Could you check a few things on this model? Use its own coordinates, in mm. Face numbers are marked on the shaded views. Give positions to 0.01 mm unless a question says otherwise; leave off trailing zeros. Loops run counter-clockwise (first coordinate to the right, second up) from the corner with the lowest first, then second, coordinate; pieces in that order, holes last. Notation, with made-up numbers: (65, 77.5) - (109, 77.5) arc R19 ccw to (109, 83.5) - close; hole circle Ø4 at (64, 0.25). An arc over 180 degrees is marked (long way). Write each question's results on one line, items separated by ' | '. Start each with the question number.
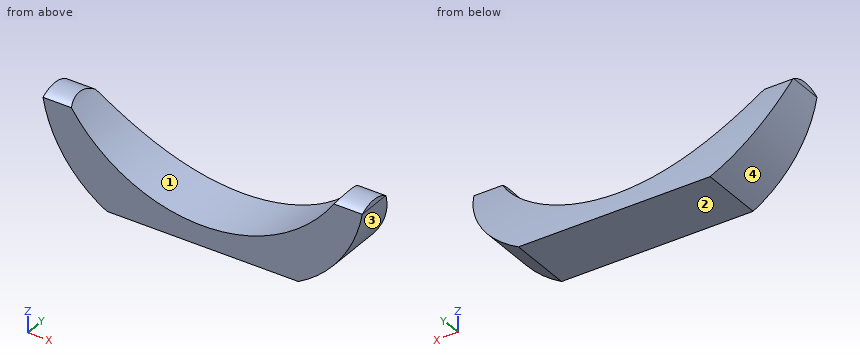
```python
from build123d import *

# Parameters (mm, degrees)
SKETCH2_W           = 500
SKETCH2_H           = 150
BOSS_EXTRUDE1_DEPTH = 100
CUT_EXTRUDE1_DEPTH  = 540
SKETCH5_R           = 249.318658331
CUT_EXTRUDE2_DEPTH  = 560
CUT_EXTRUDE3_DEPTH  = 560


with BuildPart() as part:
    # Sketch2 → Boss-Extrude1 (new body)
    with BuildSketch(Plane(origin=(0, 0, 0), x_dir=(1, 0, 0), z_dir=(0, 1, 0))):
        with Locations((96.358792185, 13.36589698)):
            Rectangle(SKETCH2_W, SKETCH2_H)
    extrude(amount=BOSS_EXTRUDE1_DEPTH)

    # Sketch4 → Cut-Extrude1 (cut)
    with BuildSketch(Plane.ZY.offset(153.641207815)):
        with BuildLine():
            Line((-88.36589698, 100), (61.63410302, 100))
            Line((61.63410302, 100), (61.63410302, 50))
            Line((61.63410302, 50), (61.63410302, 0))
            Line((61.63410302, 0), (51.789240426, 0))
            ThreePointArc((51.789240426, 0), (60.017726044, 27.945379527), (50.617731539, 55.518778225))
            ThreePointArc((50.617731539, 55.518778225), (-17.284897104, 82.724872852), (-88.36589698, 100))
        make_face()
    extrude(amount=-CUT_EXTRUDE1_DEPTH, mode=Mode.SUBTRACT)

    # Sketch5 → Cut-Extrude2 (cut)
    with BuildSketch(Plane(origin=(0, 100, 0), x_dir=(-1, 0, 0), z_dir=(0, -1, 0))):
        with Locations((-96.358792185, -192.841012905)):
            Circle(SKETCH5_R)
    extrude(amount=CUT_EXTRUDE2_DEPTH, mode=Mode.SUBTRACT)

    # Sketch6 → Cut-Extrude3 (cut)
    with BuildSketch(Plane(origin=(0, 100, 0), x_dir=(-1, 0, 0), z_dir=(0, -1, 0))):
        with BuildLine():
            Line((-246.358792185, 88.36589698), (-346.358792185, 88.36589698))
            Line((-346.358792185, 88.36589698), (-346.358792185, -51.789240426))
            ThreePointArc((-346.358792185, -51.789240426), (-312.212496259, 29.599868023), (-246.358792185, 88.36589698))
        make_face()
        with BuildLine():
            Line((53.641207815, 88.36589698), (153.641207815, 88.36589698))
            Line((153.641207815, 88.36589698), (153.641207815, -51.789240426))
            ThreePointArc((153.641207815, -51.789240426), (119.49491189, 29.599868023), (53.641207815, 88.36589698))
        make_face()
    extrude(amount=CUT_EXTRUDE3_DEPTH, mode=Mode.SUBTRACT)


solid = part.part
```
Q1. I want a section at D-D, the plane x = 5. List the corners of the cut face in (y, z) for me, then the cut area to 3 significant figures.
Q2. I'm going to push flat-ended pins straight in: pin 1 Ø1.5 at (x, y) = (-94.5, 24) entering from -Z; pin 2 Ø6 at (y, z) = (43.5, 8.5) entering from -X; pin 3 Ø5 at (y, z) = (40.5, -68.5) entering from +X. Where does each tip first touch, or does it pass through?
Q3. I want a section at B-B, the plane y = 36. List the corners of the cut face in (x, z) for me.
Q4. I want a section at C-C, the plane z = -23.5. List the corners of the cut face in (x, y) for me.
Q5. I need wall thicknesses on L1, parallel to X at y = 24.5, z = 44.5; L2, parallel to X at y = 75, z = -3.5; L3, parallel to X at y = 87, z = -69.5. Which ranges of each line are inside material? Lowest first, please. Write a range as from..to.
Q6. I want a section at A-A, the plane z = 30. List the corners of the cut face in (x, y) for me.
Q7. If we mould it in two halves opening along X, with no side actions, what happens to the marked faces 1, 2, 3 and 4? For each: +X half, -X half, draft (parallel to the pull), parting line (faces both ways), or undercut.
Conclusion:
1) outline: (0, -88.37) - (100, -88.37) arc R513.17 ccw to (89.19, -39.14) - (0, -39.14) - close | area: 4,680 mm^2
2) pin 1: z = -59.09 | pin 2: x = -142.07 | pin 3: x = 278.73
3) outline: (-153.64, 51.79) arc R200 ccw to (-53.64, -88.37) - (246.36, -88.37) arc R200 ccw to (346.36, 51.79) - (346.36, 59.17) - (306.81, 59.17) arc R249.32 cw to (-114.1, 59.17) - (-153.64, 59.17) - close
4) outline: (-123.68, 0) - (-27.56, 0) - (-27.56, 84.67) - (-123.68, 84.67) - close; (220.28, 0) - (316.4, 0) - (316.4, 84.67) - (220.28, 84.67) - close
5) L1: -152.21..-104.03, 296.75..344.93 | L2: -135.26..-57.3, 250.01..327.98 | L3: -81.77..274.48
6) outline: (-148.52, 0) - (-92.43, 0) - (-92.43, 64.98) - (-148.52, 64.98) - close; (285.15, 0) - (341.24, 0) - (341.24, 64.98) - (285.15, 64.98) - close
7) face 1: undercut | face 2: draft | face 3: +X half | face 4: -X half
